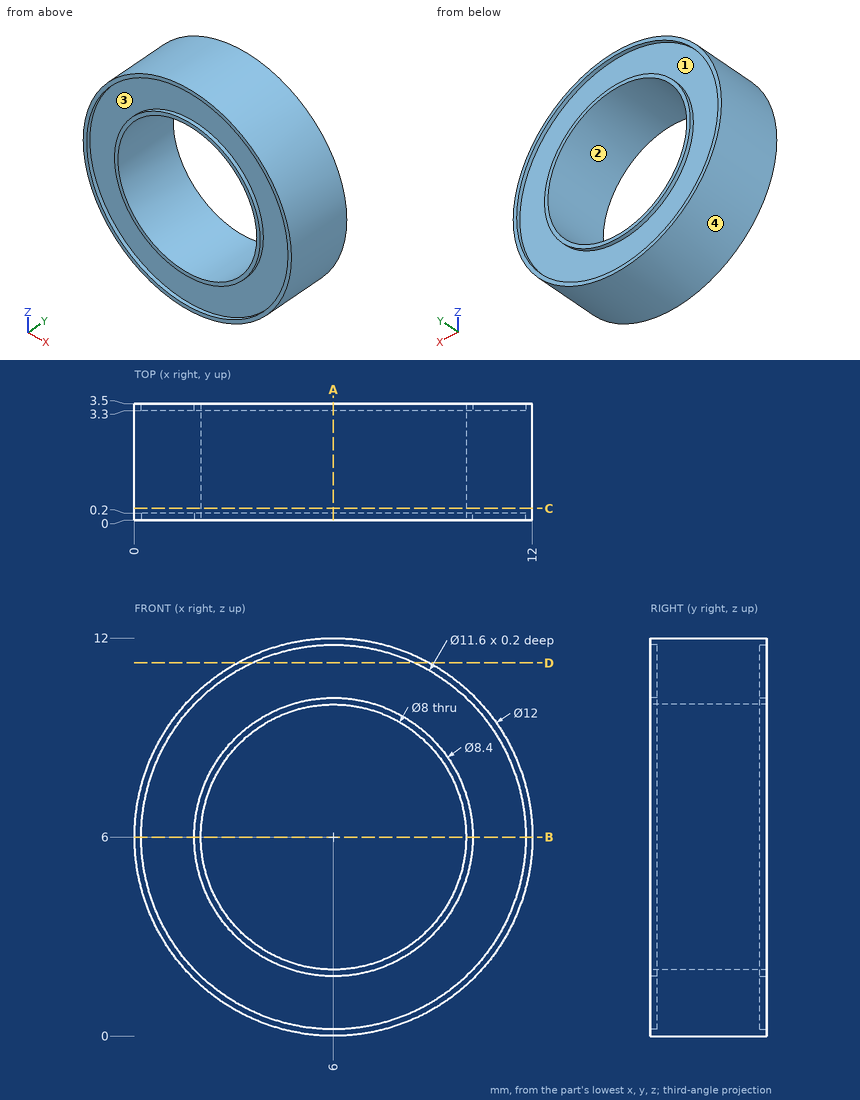
Part print with two shaded views. Sizes in mm from the minimum x, y, z corner. A direction names the side the tool comes from. Coordinates: 2 decimals unless noted, no trailing zeros. Order: outer loops, then holes, each group sorted by start corner. A loop starts at its lowest first (then second) coordinate and runs counter-clockwise, first axis right, second up. Notation, with made-up numbers: (7, 80) - (50, 80) arc R25 ccw to (50, 112) - close; hole circle Ø5 at (-40, 21.25). An arc over 180 degrees is marked (long way). Write item = value, one per line. Start each with the question number.
1) Saw through at A-A on x = 6. Write the cut outline in (y, z).
2) Two-plate mould, pull along X, no slides. Class the marked faces 3 and 4: pulls with the +X half, pulls with the -X half, needs draft (parallel to the pull), parting line crosses it, or undercut.
3) Saw through at C-C on y = 0.35. Write the cut outline in (x, z).
4) Wall check: line 1 along Z through (x, y) = (6, 0.1); line 2 along Z through (x, y) = (6, 1.1). Give the ranges that are in metal, low to high. Write a range as from..to.
5) Saw through at B-B on z = 6. Write the cut outline in (x, y), then the cut area to 3 significant figures.
6) 3-axis set-ups, long thin cutter, end or side, ignore diameter. For the marked faces 1 and 2: which of +Z, -Z, +X, -X, +Y, -Y reach the whole face in a straight line?
7) Flat gauge pin, fed straight in: pin 1 Ø1 at (y, z) = (0.5, 10) entering from -X. Where does the tip first touch, or does it go through?
8) Saw through at D-D on z = 11.25. Write the cut outline in (x, y), then the cut area to 3 significant figures.
From the geometry:
q1.outline = (0, 0) - (3.5, 0) - (3.5, 0.2) - (3.3, 0.2) - (3.3, 1.8) - (3.5, 1.8) - (3.5, 2) - (0, 2) - (0, 1.8) - (0.2, 1.8) - (0.2, 0.2) - (0, 0.2) - close; (0, 10) - (3.5, 10) - (3.5, 10.2) - (3.3, 10.2) - (3.3, 11.8) - (3.5, 11.8) - (3.5, 12) - (0, 12) - (0, 11.8) - (0.2, 11.8) - (0.2, 10.2) - (0, 10.2) - close
q2.face_3 = undercut
q2.face_4 = parting line crosses it
q3.outline = circle Ø12 at (6, 6); hole circle Ø8 at (6, 6)
q4.line_1 = 0..0.2, 1.8..2, 10..10.2, 11.8..12
q4.line_2 = 0..2, 10..12
q5.outline = (0, 0) - (0.2, 0) - (0.2, 0.2) - (1.8, 0.2) - (1.8, 0) - (2, 0) - (2, 3.5) - (1.8, 3.5) - (1.8, 3.3) - (0.2, 3.3) - (0.2, 3.5) - (0, 3.5) - close; (10, 0) - (10.2, 0) - (10.2, 0.2) - (11.8, 0.2) - (11.8, 0) - (12, 0) - (12, 3.5) - (11.8, 3.5) - (11.8, 3.3) - (10.2, 3.3) - (10.2, 3.5) - (10, 3.5) - close
q5.area = 12.7 mm^2
q6.face_1 = +Y
q6.face_2 = +Y, -Y
q7.pin_1 = 1.13
q8.outline = (3.1, 0) - (3.53, 0) - (3.53, 0.2) - (8.47, 0.2) - (8.47, 0) - (8.9, 0) - (8.9, 3.5) - (8.47, 3.5) - (8.47, 3.3) - (3.53, 3.3) - (3.53, 3.5) - (3.1, 3.5) - close
q8.area = 18.4 mm^2
